Answer from the drawing. Dimensions are ordinates in mm from the lowest x, y and z of the part. Coordinates: 2 decimals unless noted, no trailing zeros. Write each loop counter-clockwise with the first axis right and the second up, starting at its lowest first coordinate (ties: lowest second). Pieces come first, ordered by that corner, then holes.
(1) The part is cut by section B-B, the plane x = 80. Determine the outline of the cut face in (y, z), and give its area (3 significant figures).
(2) Given pin 1 (4 mm diameter, centred on x = 487, y = 11, fed in from -Z), flat-ended and moving along its own axis, determine where the tip first touches the part or whether it passes through.
(3) The part is cut by section A-A, the plane z = 80. Determine the outline of the cut face in (x, y), and give its area (3 significant figures).
(4) Straight lines are drawn through the part: line 1 along Z through (x, y) = (80, 15); line 2 along X through (y, z) = (3, 91); line 3 along X through (y, z) = (2, 64.5). For each, find the intervals that lie inside material, in ascending order.
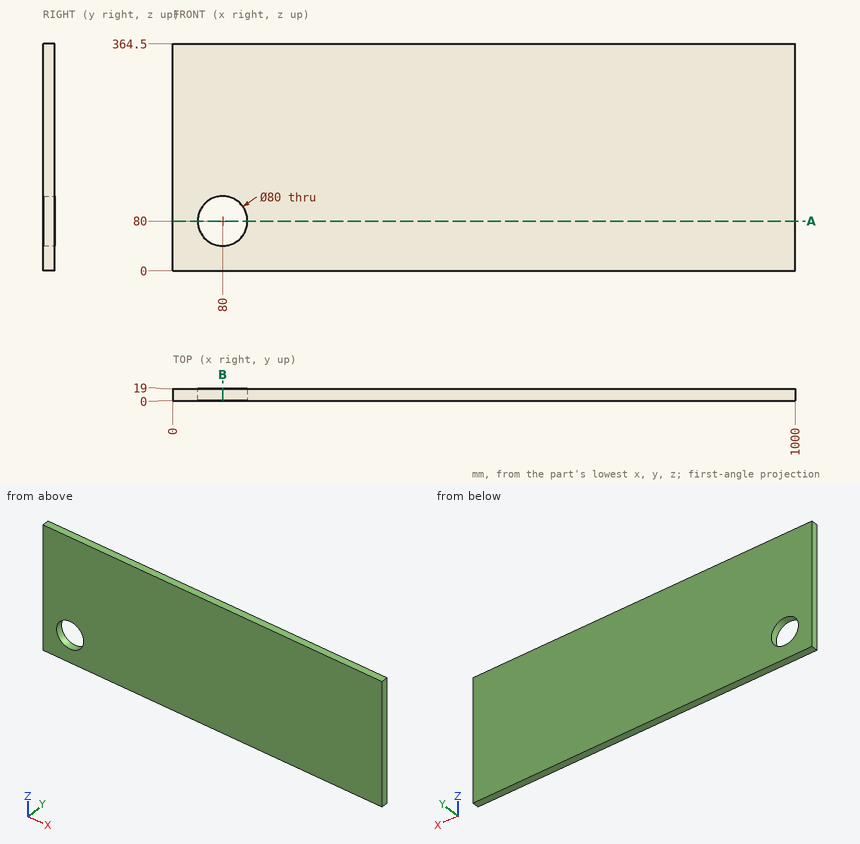
Computed:
1. outline: (0, 0) - (19, 0) - (19, 40) - (0, 40) - close; (0, 120) - (19, 120) - (19, 364.5) - (0, 364.5) - close
1. area: 5,410 mm2
2. pin 1: stops at z = 0
3. outline: (0, 0) - (40, 0) - (40, 19) - (0, 19) - close; (120, 0) - (1000, 0) - (1000, 19) - (120, 19) - close
3. area: 17,500 mm2
4. line 1: z = 0 to 40, 120 to 364.5
4. line 2: x = 0 to 41.54, 118.46 to 1000
4. line 3: x = 0 to 43.13, 116.87 to 1000
